```python
from build123d import *

# Parameters (mm, degrees)
SKETCH1_W                          = 21
SKETCH1_H                          = 26
BOSS_EXTRUDE1_DEPTH                = 2
FILLET1_R                          = 2
SKETCH2_R                          = 5
BOSS_EXTRUDE2_DEPTH                = 5
F_3_0_3_DIAMETER_HOLE1_D           = 3
F_3_0_3_DIAMETER_HOLE1_CSINK_D     = 3.05
F_3_0_3_DIAMETER_HOLE1_CSINK_ANGLE = 90


with BuildPart() as part:
    # Sketch1 → Boss-Extrude1 (new body)
    with BuildSketch(Plane(origin=(0, 0, 0), x_dir=(1, 0, 0), z_dir=(0, 1, 0))):
        Rectangle(SKETCH1_W, SKETCH1_H)
    extrude(amount=BOSS_EXTRUDE1_DEPTH)

    # Fillet1
    fillet1_edges = [part.edges().sort_by_distance(p)[0] for p in [
        (10.5, 1, 13),
        (-10.5, 1, 13),
        (-10.5, 1, -13),
        (10.5, 1, -13),
    ]]
    fillet(fillet1_edges, radius=FILLET1_R)

    # Sketch2 → Boss-Extrude2 (add)
    with BuildSketch(Plane(origin=(0, 2, 0), x_dir=(1, 0, 0), z_dir=(0, 1, 0))):
        with Locations(Location((0, 3, 0), (0, 0, 270))):
            Circle(SKETCH2_R)
    extrude(amount=BOSS_EXTRUDE2_DEPTH)

    # Ø3.0 (3) Diameter Hole1 (through all)
    with Locations(Plane(origin=(0, 2, 0), x_dir=(1, 0, 0), z_dir=(0, 1, 0))):
        with Locations((-7.5, -11), (7.5, -11)):
            CounterSinkHole(F_3_0_3_DIAMETER_HOLE1_D / 2, F_3_0_3_DIAMETER_HOLE1_CSINK_D / 2, counter_sink_angle=F_3_0_3_DIAMETER_HOLE1_CSINK_ANGLE)


solid = part.part
```
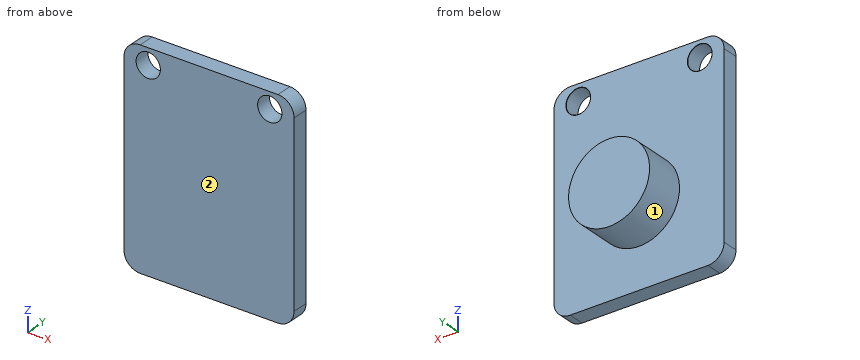
Source: CAD feature listing. Evaluate the final solid. Frame: model axes, mm. Face numbers are marked on the shaded views. A direction names the side the tool comes from. Give positions to 0.01 mm unless a question says otherwise; leave off trailing zeros. Write each loop counter-clockwise with the first axis right and the second up, starting at its lowest first coordinate (ties: lowest second). Pieces come first, ordered by that corner, then holes.
1. Section query A-A (z = -3). Return the cut outline in (x, y).
2. Material intervals for line 1 along X through (y, z) = (0.5, 11); line 2 along Z through (x, y) = (-7.5, 1.5); line 3 along Y through (x, z) = (-6, 0), sorted ascending.
3. First-contact query: pin 1 (4 mm diameter, centred on x = 7.5, z = 11, fed in from +Y). Flat tip, straight axial feed; report the tip coordinate or a pass-through.
4. Section query D-D (x = 0). Return the cut outline in (y, z), then the cut area to 3 significant figures.
5. Section query C-C (y = 1). Return the cut outline in (x, z).
6. Access query for the marked faces 1 and 2. Directions: +Z, -Z, +X, -X, +Y, -Y. A direction counts if a zero-diameter tool reaches every point of the face in a straight line with its end or side. Return the directions, or none.
7. Section query B-B (x = 7.5). Return the cut outline in (y, z) (3 decimals), then the cut area to 3 significant figures.
Output values:
1. outline: (-10.5, 0) - (10.5, 0) - (10.5, 2) - (5, 2) - (5, 7) - (-5, 7) - (-5, 2) - (-10.5, 2) - close
2. line 1: x = -10.5 to -9, -6 to 6, 9 to 10.5
2. line 2: z = -13 to 9.5, 12.5 to 13
2. line 3: y = 0 to 2
3. pin 1: stops at y = 2
4. outline: (0, -13) - (2, -13) - (2, -8) - (7, -8) - (7, 2) - (2, 2) - (2, 13) - (0, 13) - close
4. area: 102 mm2
5. outline: (-10.5, -11) arc R2 ccw to (-8.5, -13) - (8.5, -13) arc R2 ccw to (10.5, -11) - (10.5, 11) arc R2 ccw to (8.5, 13) - (-8.5, 13) arc R2 ccw to (-10.5, 11) - close; hole circle Ø3 at (-7.5, 11); hole circle Ø3 at (7.5, 11)
6. face 1: +Y
6. face 2: +Z, -Z, +X, -X, -Y
7. outline: (0, -13) - (2, -13) - (2, 9.475) - (1.975, 9.5) - (0, 9.5) - close; (0, 12.5) - (1.975, 12.5) - (2, 12.525) - (2, 13) - (0, 13) - close
7. area: 46.0 mm2
